Part model, mm, in its own coordinate system. Coordinates: 2 decimals unless noted, no trailing zeros. Loops run counter-clockwise (first coordinate to the right, second up) from the corner with the lowest first, then second, coordinate; pieces in that order, holes last. Notation, with made-up numbers: M -18.75,46 L 21.25,46 A34 ccw 21.25,78 Z; hole C 85,61.5 d7. An arc over 180 degrees is marked long. Use a Markdown table: item, result. Add a question column.
1) Band-saw the part on A-A (z = 29.5). List the corners of the cut face in (x, y) (3 decimals).
2) Band-saw the part on C-C (y = -4.75). List the corners of the cut face in (x, z).
3) Pin check, flat tips, straight feed: pin 1 Ø6 at (x, y) = (48, -3.5) entering from -Z; pin 2 Ø4 at (x, y) = (35.56, -6.35) entering from +Z. Stop position of each tip, or through.
4) Wall check: probe 1 along X at (y, z) = (-4.25, 29); probe 2 along Y at (x, z) = (35.56, 27) (3 decimals); probe 3 along X at (y, z) = (-4, 18). Give the ranges that are in metal, low to high. Write a range as from..to.
5) Band-saw the part on B-B (x = 8). List the corners of the cut face in (y, z).
6) Band-saw the part on D-D (x = 35.56). List the corners of the cut face in (y, z) (3 decimals).
7) Pull direction Y, two halves, no side cores. Call faces 1 (the flat face through (35, -12.7, 22)), 2 (the cylindrical face through (32.39, -6.21, 27.73)), 3 (the flat face through (0, -6, 15)): released by +Y, released by -Y, zero draft, split by the parting line, or undercut.
from build123d import *

# Parameters (mm, degrees)
F1_DEPTH    = 12.7
F2_R        = 3.175
F3_DEPTH    = 35.561
F4_R        = 3.175
F5_DEPTH    = 15.8764097817
F6_T1_DEPTH = 38.1


# Not quite as in the source:
# - a fillet or chamfer that OpenCascade refuses, or shapes differently, is made with other operations: its cross-section is extruded or revolved along the edge and cut away or added


with BuildPart() as f1:
    # F0 (on Front) → F1 (new body)
    with BuildSketch(Plane.XZ):
        with BuildLine():
            Line((0, 35.56), (0, 0))
            Line((0, 0), (15.621, 0))
            ThreePointArc((15.621, 0), (35.56, 19.939), (55.499, 0))
            Line((55.499, 0), (71.12, 0))
            Line((71.12, 0), (71.12, 35.56))
            Line((71.12, 35.56), (0, 35.56))
        make_face()
    extrude(amount=F1_DEPTH)

    # F2 (on face) → F3 (cut, through all)
    with BuildSketch(Plane.XY.offset(35.56)):
        with Locations((6.985, -6.35)):
            Circle(F2_R)
        with Locations((64.135, -6.35)):
            Circle(F2_R)
    extrude(amount=-F3_DEPTH, mode=Mode.SUBTRACT)

    # F4 (on face) → F5 (cut, through all)
    with BuildSketch(Plane.XY.offset(35.56)):
        with Locations((35.56, -6.35)):
            Circle(F4_R)
    extrude(amount=-F5_DEPTH, mode=Mode.SUBTRACT)

    # F6: fillet of radius 5.08 on 2 edges, made by hand

    # F6_s2 → F6_t1 (cut)
    with BuildSketch(Plane.XZ.offset(-12.7)):
        with BuildLine():
            ThreePointArc((0, 30.48), (1.4878975516, 34.0721024484), (5.08, 35.56))
            Line((5.08, 35.56), (0, 35.56))
            Line((0, 35.56), (0, 30.48))
        make_face()
        with BuildLine():
            ThreePointArc((66.04, 35.56), (69.6321024484, 34.0721024484), (71.12, 30.48))
            Line((71.12, 30.48), (71.12, 35.56))
            Line((71.12, 35.56), (66.04, 35.56))
        make_face()
    extrude(amount=F6_T1_DEPTH, mode=Mode.SUBTRACT)


solid = f1.part
Entries:
| question | item | result |
|---|---|---|
| 1 | outline | M 0,-12.7 L 71.12,-12.7 L 71.12,0 L 0,0 Z; hole C 6.985,-6.35 d6.35; hole C 35.56,-6.35 d6.35; hole C 64.135,-6.35 d6.35 |
| 2 | outline | M 0,0 L 4.24,0 L 4.24,35.49 A5.08 ccw 0,30.48 Z; M 9.73,0 L 15.62,0 A19.94 cw 32.82,19.75 L 32.82,35.56 L 9.73,35.56 Z; M 38.3,19.75 A19.94 cw 55.5,0 L 61.39,0 L 61.39,35.56 L 38.3,35.56 Z; M 66.88,0 L 71.12,0 L 71.12,30.48 A5.08 ccw 66.88,35.49 Z |
| 3 | pin 1 | z = 12.62 |
| 3 | pin 2 | through |
| 4 | probe 1 | 0..4.6, 9.37..33.18, 37.94..61.75, 66.52..71.12 |
| 4 | probe 2 | -12.7..-9.525, -3.175..0 |
| 4 | probe 3 | 0..4.85, 9.12..26.98, 44.14..62, 66.27..71.12 |
| 5 | outline | M -12.7,0 L -9.36,0 L -9.36,35.56 L -12.7,35.56 Z; M -3.34,0 L 0,0 L 0,35.56 L -3.34,35.56 Z |
| 6 | outline | M -12.7,19.939 L -9.525,19.939 L -9.525,35.56 L -12.7,35.56 Z; M -3.175,19.939 L 0,19.939 L 0,35.56 L -3.175,35.56 Z |
| 7 | face 1 | released by -Y |
| 7 | face 2 | undercut |
| 7 | face 3 | zero draft |
